Source: CAD feature listing. Evaluate the final solid. Frame: model axes, mm. Face numbers are marked on the shaded views. A direction names the side the tool comes from. Round coordinates to 2 decimals unless told otherwise and drop trailing zeros. Order: outer loops, then holes, each group sorted by start corner. A loop starts at its lowest first (then second) coordinate and runs counter-clockwise, first axis right, second up. Notation, with made-up numbers: (25.25, -24) -> (33.25, -24) arc R36 ccw to (33.25, 15) -> close; hole circle Ø3 at (56.25, -2.5). An arc over 180 degrees is marked (long way). One line per item, written item: value. Start each with the question number.
1) Pin query (flat end, axial travel): P1, Ø2.5, axis at x = 4, z = 1.5, coming from the +Y side. Return the tip coordinate at first contact, or that it passes through.
2) Ray query, L1, parallel to Z at x = 9.75, y = 22.86; L2, parallel to X at y = 23, z = 1; L3, parallel to Y at x = -2.5, z = 3.25. Return the intervals inside material, ascending.
3) Mould query, pull axis X, two halves, no side actions, for the marked faces 1, 2 and 3. Classes: pulls with the +X half, pulls with the -X half, needs draft (parallel to the pull), parting line crosses it, or undercut.
4) Reachability of the marked faces 4 and 5 from +Z, -Z, +X, -X, +Y, -Y: full face, straight path, thin tool, end or side. Return the list, or none.
5) Section B-B (x = -7). Return the cut outline in (y, z).
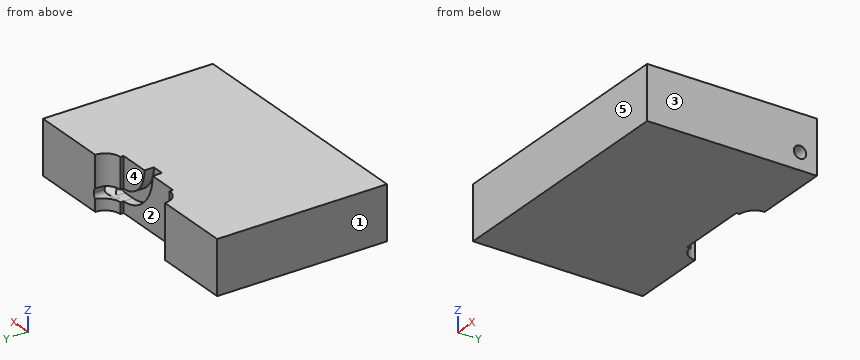
```python
from build123d import *

# Parameters (mm, degrees)
SKETCH1_W               = 38.1
SKETCH1_H               = 8.001
BOSS_EXTRUDE1_DEPTH     = 25.4
CUT_EXTRUDE1_DEPTH      = 25.4
CUT_EXTRUDE2_DEPTH      = 31.267193568
CUT_EXTRUDE2_DEPTH_BACK = 1.905
SKETCH5_R               = 0.9271
CUT_EXTRUDE3_DEPTH      = 12.7
SKETCH6_W               = 10.795
SKETCH6_H               = 8.001
CUT_EXTRUDE4_DEPTH      = 0.508


with BuildPart() as part:
    # Sketch1 → Boss-Extrude1 (new body)
    with BuildSketch(Plane(origin=(0, 0, 0), x_dir=(1, 0, 0), z_dir=(0, 1, 0))):
        Rectangle(SKETCH1_W, SKETCH1_H)
    extrude(amount=BOSS_EXTRUDE1_DEPTH)

    # Sketch2 → Cut-Extrude1 (cut)
    with BuildSketch(Plane(origin=(0, 0, -4.0005), x_dir=(-1, 0, 0), z_dir=(0, 0, -1))):
        with BuildLine():
            Line((5.3975, 23.1775), (-5.3975, 23.1775))
            ThreePointArc((-5.3975, 23.1775), (-7.62, 25.4), (-5.3975, 27.6225))
            Line((-5.3975, 27.6225), (5.3975, 27.6225))
            ThreePointArc((5.3975, 27.6225), (7.62, 25.4), (5.3975, 23.1775))
        make_face()
    extrude(amount=-CUT_EXTRUDE1_DEPTH, mode=Mode.SUBTRACT)

    # Sketch4 → Cut-Extrude2 (cut, two sides: drawn at the far end of the back side and taken through both)
    with BuildSketch(Plane(origin=(0, 23.1775, 0), x_dir=(1, 0, 0), z_dir=(0, 1, 0)).offset(-CUT_EXTRUDE2_DEPTH_BACK)):
        with BuildLine():
            Line((0.8255, -4.0005), (-0.9525, -4.0005))
            ThreePointArc((-0.9525, -4.0005), (0.907371939, 0.489628061), (5.3975, 2.3495))
            Line((5.3975, 2.3495), (7.14375, 2.3495))
            ThreePointArc((7.14375, 2.3495), (7.705016008, 2.117016008), (7.9375, 1.55575))
            Line((7.9375, 1.55575), (7.9375, 1.36525))
            ThreePointArc((7.9375, 1.36525), (7.705016008, 0.803983992), (7.14375, 0.5715))
            Line((7.14375, 0.5715), (5.3975, 0.5715))
            ThreePointArc((5.3975, 0.5715), (2.164607796, -0.767607796), (0.8255, -4.0005))
        make_face()
    extrude(amount=CUT_EXTRUDE2_DEPTH + CUT_EXTRUDE2_DEPTH_BACK, mode=Mode.SUBTRACT)

    # Sketch5 → Cut-Extrude3 (cut)
    with BuildSketch(Plane(origin=(19.05, 0, 0), x_dir=(0, 0, -1), z_dir=(1, 0, 0))):
        with Locations((1.4605, 22.86)):
            Circle(SKETCH5_R)
    extrude(amount=-CUT_EXTRUDE3_DEPTH, mode=Mode.SUBTRACT)

    # Sketch6 → Cut-Extrude4 (cut)
    with BuildSketch(Plane(origin=(0, 23.1775, 0), x_dir=(1, 0, 0), z_dir=(0, 1, 0))):
        Rectangle(SKETCH6_W, SKETCH6_H)
    extrude(amount=-CUT_EXTRUDE4_DEPTH, mode=Mode.SUBTRACT)


solid = part.part
```
Findings:
1. P1: y = 22.67
2. L1: -4 to -2.39, -0.53 to 4
2. L2: -19.05 to -5.4, 5.4 to 19.05
2. L3: 0 to 22.67
3. face 1: pulls with the -X half
3. face 2: undercut
3. face 3: pulls with the +X half
4. face 4: +Z, -Z, +Y
4. face 5: +Z, -Z, +X, -X, -Y
5. outline: (0, -4) -> (23.86, -4) -> (23.86, 4) -> (0, 4) -> close
